Geometry: final body of the model. Coordinates: model frame, mm. A direction names the side the tool comes from. Give positions to 0.01 mm unless a question says otherwise; leave off trailing zeros. Order: outer loops, then holes, each group sorted by start corner. A loop starts at its lowest first (then second) coordinate and runs counter-clockwise, first axis right, second up. Notation, with made-up numbers: (47, -28) -> (95, -28) arc R28 cw to (95, 5) -> close; hole circle Ø9 at (48, -20). An arc over 180 degrees is marked (long way). Answer in a Markdown table with one row per item. Add a question column.
Q1. Line query: line 1 along X through (y, z) = (-1.65, 29.5); line 2 along X through (y, z) = (-0.85, 34.5); line 3 along X through (y, z) = (-0.15, 32.5). Output: solid intervals per line, ascending. Write a range as from..to.
Q2. Pull-direction query (Z, two-part tool) for faces 4 (the face through (22.196, -1.565, 6.824)), 5 (the face through (-10, -2, 22.073)), 6 (the face through (-33, 0, 15)), 7 (the face through (-1.36, -1.57, -12.58)); classes: +Z half, -Z half, draft (parallel to the pull), parting line (faces both ways), or undercut.
Q3. Contact query for flat-ended pins moving along their axis: P1, Ø1, axis at x = -42, y = -1.5, coming from the +Z side; P2, Ø1.6, axis at y = -1, z = 17.5, coming from the +X side. Output: stop coordinate, or through.
Q4. Cut plane B-B on y = -2.6. Count the separate pieces of the cut face and the enclosed holes in it, and give its area (3 significant figures).
Q5. Set-up query: faces 1 (the face through (-17.038, -1.61, 14.912)), 2 (the face through (-67.09, -1.61, 32.24)), 3 (the face through (-6.405, -1.565, 27.345)). Return all of +Z, -Z, +X, -X, +Y, -Y with unobstructed straight access to the full face (end or side cutting, diameter ignored); none if empty.
Q6. Cut plane C-C on x = -12. Return the cut outline in (y, z) (3 decimals), and give its area (3 significant figures).
Q7. Cut plane D-D on z = 24. Return the cut outline in (x, y) (3 decimals).
Q8. Cut plane A-A on x = 0. Return the cut outline in (y, z) (3 decimals), and give its area (3 significant figures).
from build123d import *

# Parameters (mm, degrees)
F0_R        = 2.3495
F0_R_2      = 4.3561
F1_DEPTH    = 3.175
F2_T1_DEPTH = 8.6796915338
F2_T3_DEPTH = 9.317688033
F3_R        = 3.048
F4_R        = 3.175
F5_R        = 1.524


# Not quite as in the source:
# - a fillet or chamfer that OpenCascade refuses, or shapes differently, is made with other operations: its cross-section is extruded or revolved along the edge and cut away or added


with BuildPart() as f1:
    # F0 (on Front) → F1 (new body)
    with BuildSketch(Plane.XZ):
        with BuildLine():
            Line((-17.907, 13.9954), (-17.907, 22.0726))
            Line((-17.907, 22.0726), (-5.461, 22.0726))
            ThreePointArc((-5.461, 22.0726), (4.064, 31.5976), (-5.461, 41.1226))
            ThreePointArc((-5.461, 41.1226), (-12.1961920908, 38.3327920908), (-14.986, 31.5976))
            Line((-14.986, 31.5976), (-67.945, 31.5976))
            ThreePointArc((-67.945, 31.5976), (-70.7348079092, 38.3327920908), (-77.47, 41.1226))
            ThreePointArc((-77.47, 41.1226), (-86.7805213206, 33.6075297847), (-81.3993425959, 22.9208556933))
            Line((-81.3993425959, 22.9208556933), (-5.461, -11.4685135998))
            ThreePointArc((-5.461, -11.4685135998), (-0.6838491315, -12.6351736228), (4.191, -11.9885578365))
            Line((4.191, -11.9885578365), (4.191, -9.8147056722))
            Line((4.191, -9.8147056722), (-2.5137480378, -7.5958588588))
            ThreePointArc((-2.5137480378, -7.5958588588), (-7.5958588588, 2.5137480378), (2.5137480378, 7.5958588588))
            Line((2.5137480378, 7.5958588588), (15.2275267548, 3.3884035996))
            ThreePointArc((15.2275267548, 3.3884035996), (22.2730028192, 7.0612251677), (18.3941407903, 13.9954))
            Line((18.3941407903, 13.9954), (-17.907, 13.9954))
        make_face()
        with Locations((16.9672, 8.6452202067)):
            Circle(F0_R, mode=Mode.SUBTRACT)
        with Locations((-77.47, 31.5976)):
            Circle(F0_R_2, mode=Mode.SUBTRACT)
        with Locations((-5.461, 31.5976)):
            Circle(F0_R_2, mode=Mode.SUBTRACT)
    extrude(amount=F1_DEPTH)

    # F2: fillet of radius 1.524 on 2 edges, made by hand

    # F2_s2 → F2_t1 (cut)
    with BuildSketch(Plane.XZ.offset(-2.7523457669)):
        with BuildLine():
            ThreePointArc((3.1458091501, -9.4688137202), (3.9023706215, -10.0232116691), (4.191, -10.915643979))
            Line((4.191, -10.915643979), (4.191, -9.8147056722))
            Line((4.191, -9.8147056722), (3.1458091501, -9.4688137202))
        make_face()
    extrude(amount=F2_T1_DEPTH, mode=Mode.SUBTRACT)

    # F2_s4 → F2_t3 (cut)
    with BuildSketch(Plane.XZ.offset(-3.0713440165)):
        with BuildLine():
            ThreePointArc((4.191, -10.8324529742), (3.8589330034, -11.7821222406), (3.0074413182, -12.3179413481))
            ThreePointArc((3.0074413182, -12.3179413481), (3.6030210464, -12.1669053498), (4.191, -11.9885578365))
            Line((4.191, -11.9885578365), (4.191, -10.8324529742))
        make_face()
    extrude(amount=F2_T3_DEPTH, mode=Mode.SUBTRACT)

    # F3
    f3_edges = [f1.edges().sort_by_distance(p)[0] for p in [
        (-17.907, -1.5875, 22.0726),
        (-17.907, -1.5875, 13.9954),
    ]]
    fillet(f3_edges, radius=F3_R)

    # F4
    f4_edges = [f1.edges().sort_by_distance(p)[0] for p in [
        (-67.945, -1.5875, 31.5976),
        (-14.986, -1.5875, 31.5976),
    ]]
    fillet(f4_edges, radius=F4_R)

    # F5
    f5_edges = [f1.edges().sort_by_distance(p)[0] for p in [
        (18.394141, -1.5875, 13.9954),
    ]]
    fillet(f5_edges, radius=F5_R)


solid = f1.part
Completed:
| question | item | result |
|---|---|---|
| 1 | line 1 | x = -86.76..-81.29, -73.65..-9.28, -1.64..3.83 |
| 1 | line 2 | x = -86.54..-80.72, -74.22..-68.4, -14.53..-8.71, -2.21..3.61 |
| 1 | line 3 | x = -86.95..-81.73, -73.21..-67.39, -15.54..-9.72, -1.2..4.02 |
| 2 | face 4 | parting line |
| 2 | face 5 | undercut |
| 2 | face 6 | draft |
| 2 | face 7 | -Z half |
| 3 | P1 | stops at z = 31.6 |
| 3 | P2 | stops at x = -17.89 |
| 4 | separate pieces | 1 |
| 4 | enclosed holes | 3 |
| 4 | area | 2,370 mm² |
| 5 | face 1 | +X, +Y, -Y |
| 5 | face 2 | +Z, +Y, -Y |
| 5 | face 3 | +Y, -Y |
| 6 | outline | (-3.175, -8.507) -> (0, -8.507) -> (0, 13.995) -> (-3.175, 13.995) -> close; (-3.175, 22.073) -> (0, 22.073) -> (0, 38.523) -> (-3.175, 38.523) -> close |
| 6 | area | 124 mm² |
| 7 | outline | (-83.215, -3.175) -> (0.284, -3.175) -> (0.284, 0) -> (-83.215, 0) -> close |
| 8 | outline | (-3.175, -12.654) -> (0, -12.654) -> (0, -8.428) -> (-3.175, -8.428) -> close; (-3.175, 8.001) -> (0, 8.001) -> (0, 13.995) -> (-3.175, 13.995) -> close; (-3.175, 23.794) -> (0, 23.794) -> (0, 39.402) -> (-3.175, 39.402) -> close |
| 8 | area | 82.0 mm² |
